from build123d import *

# Parameters (mm, degrees)
SKETCH1_R           = 4.7625
SKETCH1_R_2         = 0.635
BOSS_EXTRUDE1_DEPTH = 2.54
SKETCH2_R           = 2.9845
CUT_EXTRUDE1_DEPTH  = 0.254
CUT_EXTRUDE2_START  = -0.254
SKETCH3_R           = 2.9845
CUT_EXTRUDE2_DEPTH  = 0.254


with BuildPart() as part:
    # Sketch1 → Boss-Extrude1 (new body)
    with BuildSketch(Plane.XY):
        Circle(SKETCH1_R)
        Circle(SKETCH1_R_2, mode=Mode.SUBTRACT)
    extrude(amount=BOSS_EXTRUDE1_DEPTH)

    # Sketch2 → Cut-Extrude1 (cut)
    with BuildSketch(Plane.XY.offset(2.54)):
        Circle(SKETCH2_R)
    extrude(amount=-CUT_EXTRUDE1_DEPTH, mode=Mode.SUBTRACT)

    # Sketch3 → Cut-Extrude2 (cut)
    with BuildSketch(Plane(origin=(0, 0, 0), x_dir=(-1, 0, 0), z_dir=(0, 0, -1)).offset(CUT_EXTRUDE2_START)):
        with Locations(Location((0, 0, 0), (0, 0, 180))):
            Circle(SKETCH3_R)
    extrude(amount=CUT_EXTRUDE2_DEPTH, mode=Mode.SUBTRACT)


solid = part.part
Read the model definition and answer for the solid it produces. Units are mm, in the model's axes. A direction names the side the tool comes from. Coordinates: 2 decimals unless noted, no trailing zeros. Loops run counter-clockwise (first coordinate to the right, second up) from the corner with the lowest first, then second, coordinate; pieces in that order, holes last. Notation, with made-up numbers: (46.25, 30.5) - (53.25, 30.5) arc R23 ccw to (53.25, 40.5) - close; hole circle Ø9 at (46.5, -11.5). An arc over 180 degrees is marked (long way). Answer in a Markdown table with one row per item.
Q1. Given P1, Ø5, axis at x = 0, y = 0, coming from the +Z side; P2, Ø1, axis at x = 0, y = 0, coming from the -Z side, each flat-ended and moving along its own axis, determine where each tip first touches the part or whether it passes through.
Here are the results:
| item | result |
|---|---|
| P1 | stops at z = 2.29 |
| P2 | passes through |
Q2. Find section C-C on x = 2.25. Write down the section's boundary in (y, z), plus the area to 3 significant figures.
Here are the results:
| item | result |
|---|---|
| outline | (-4.2, 0) - (-1.96, 0) - (-1.96, 0.25) - (1.96, 0.25) - (1.96, 0) - (4.2, 0) - (4.2, 2.54) - (1.96, 2.54) - (1.96, 2.29) - (-1.96, 2.29) - (-1.96, 2.54) - (-4.2, 2.54) - close |
| area | 19.3 mm^2 |
Q3. The mould has two halves that part along X. Classify faces 1 (the flat face through (1, -3, 0)), 2 (the cylindrical face through (-0.08, 0.63, 1.26)), 3 (the flat face through (0, -1, 0.254)), 4 (the cylindrical face through (-3.78, -2.9, 1.25)): pulls with the +X half, pulls with the -X half, needs draft (parallel to the pull), parting line crosses it, or undercut.
Here are the results:
| item | result |
|---|---|
| face 1 | needs draft |
| face 2 | undercut |
| face 3 | undercut |
| face 4 | parting line crosses it |
Q4. Find section D-D on z = 1.8. Write down the section's boundary in (x, y) (1 decimal).
Here are the results:
| item | result |
|---|---|
| outline | circle Ø9.5 at (0, 0); hole circle Ø1.3 at (0, 0) |
Q5. Straight lines are drawn through the part: line 1 along Y through (x, z) = (0, 0.15); line 2 along Y through (x, z) = (0, 1.65) (1 decimal); line 3 along Z through (x, y) = (-0.75, 2). For each, find the intervals that lie inside material, in ascending order. Write a range as [from, to].
Here are the results:
| item | result |
|---|---|
| line 1 | y = [-4.76, -2.98], [2.98, 4.76] |
| line 2 | y = [-4.8, -0.6], [0.6, 4.8] |
| line 3 | z = [0.25, 2.29] |
Q6. For faces 5 (the flat face through (0, 1, 2.286)), 6 (the flat face through (1, -3, 2.54)), determine the directions among +Z, -Z, +X, -X, +Y, -Y from which every point of the face is accessible in a straight line to the end or side of a thin tool.
Here are the results:
| item | result |
|---|---|
| face 5 | +Z |
| face 6 | +Z, +X, -X, +Y, -Y |
